from build123d import *

# Parameters (mm, degrees)
SKETCH1_R           = 4
BOSS_EXTRUDE1_DEPTH = 8.9
SKETCH2_R           = 5
BOSS_EXTRUDE2_DEPTH = 1.5
BOSS_EXTRUDE3_START = -1.5
SKETCH3_R           = 40
BOSS_EXTRUDE3_DEPTH = 3
CUT_EXTRUDE2_START  = 8.9
SKETCH5_R           = 2.2
CUT_EXTRUDE2_DEPTH  = 2
CUT_EXTRUDE3_DEPTH  = 10


with BuildPart() as part:
    # Sketch1 → Boss-Extrude1 (new body)
    with BuildSketch(Plane.XY):
        Circle(SKETCH1_R)
    extrude(amount=BOSS_EXTRUDE1_DEPTH)

    # Sketch2 → Boss-Extrude2 (add)
    with BuildSketch(Plane.XY):
        Circle(SKETCH2_R)
    extrude(amount=-BOSS_EXTRUDE2_DEPTH)

    # Sketch3 → Boss-Extrude3 (add)
    with BuildSketch(Plane.XY.offset(BOSS_EXTRUDE3_START)):
        Circle(SKETCH3_R)
    extrude(amount=-BOSS_EXTRUDE3_DEPTH)

    # Sketch5 → Cut-Extrude2 (cut)
    with BuildSketch(Plane.XY.offset(CUT_EXTRUDE2_START)):
        Circle(SKETCH5_R)
    extrude(amount=-CUT_EXTRUDE2_DEPTH, mode=Mode.SUBTRACT)

    # Sketch6 → Cut-Extrude3 (cut)
    with BuildSketch(Plane.XY):
        with BuildLine():
            Line((30.266810214, -15.165149948), (8.5033321, -2.6))
            ThreePointArc((8.5033321, -2.6), (7.973884535, -2.083913954), (7.755291283, -1.377602039))
            ThreePointArc((7.755291283, -1.377602039), (8, 0), (7.755291283, 1.377602039))
            ThreePointArc((7.755291283, 1.377602039), (7.973884535, 2.083913954), (8.5033321, 2.6))
            Line((8.5033321, 2.6), (30.266810214, 15.165149948))
            ThreePointArc((30.266810214, 15.165149948), (31.724798793, 15.379954672), (32.934114256, 14.537679256))
            ThreePointArc((32.934114256, 14.537679256), (36, 0), (32.934114256, -14.537679256))
            ThreePointArc((32.934114256, -14.537679256), (31.724798793, -15.379954672), (30.266810214, -15.165149948))
        make_face()
        with BuildLine():
            Line((2, 33.794401511), (2, 8.664101615))
            ThreePointArc((2, 8.664101615), (2.182219844, 7.947543551), (2.684607279, 7.405080285))
            ThreePointArc((2.684607279, 7.405080285), (4, 6.92820323), (5.070684004, 6.027478245))
            ThreePointArc((5.070684004, 6.027478245), (5.791664691, 5.863629597), (6.5033321, 6.064101615))
            Line((6.5033321, 6.064101615), (28.266810214, 18.629251563))
            ThreePointArc((28.266810214, 18.629251563), (29.181830852, 19.784504349), (29.057056676, 21.252939969))
            ThreePointArc((29.057056676, 21.252939969), (18, 31.176914536), (3.87705758, 35.790619225))
            ThreePointArc((3.87705758, 35.790619225), (2.542967941, 35.164459021), (2, 33.794401511))
        make_face()
        with BuildLine():
            Line((2, -33.794401511), (2, -8.664101615))
            ThreePointArc((2, -8.664101615), (2.182219844, -7.947543551), (2.684607279, -7.405080285))
            ThreePointArc((2.684607279, -7.405080285), (4, -6.92820323), (5.070684004, -6.027478245))
            ThreePointArc((5.070684004, -6.027478245), (5.791664691, -5.863629597), (6.5033321, -6.064101615))
            Line((6.5033321, -6.064101615), (28.266810214, -18.629251563))
            ThreePointArc((28.266810214, -18.629251563), (29.181830852, -19.784504349), (29.057056676, -21.252939969))
            ThreePointArc((29.057056676, -21.252939969), (18, -31.176914536), (3.87705758, -35.790619225))
            ThreePointArc((3.87705758, -35.790619225), (2.542967941, -35.164459021), (2, -33.794401511))
        make_face()
        with BuildLine():
            Line((-28.266810214, -18.629251563), (-6.5033321, -6.064101615))
            ThreePointArc((-6.5033321, -6.064101615), (-5.791664691, -5.863629597), (-5.070684004, -6.027478245))
            ThreePointArc((-5.070684004, -6.027478245), (-4, -6.92820323), (-2.684607279, -7.405080285))
            ThreePointArc((-2.684607279, -7.405080285), (-2.182219844, -7.947543551), (-2, -8.664101615))
            Line((-2, -8.664101615), (-2, -33.794401511))
            ThreePointArc((-2, -33.794401511), (-2.542967941, -35.164459021), (-3.87705758, -35.790619225))
            ThreePointArc((-3.87705758, -35.790619225), (-18, -31.176914536), (-29.057056676, -21.252939969))
            ThreePointArc((-29.057056676, -21.252939969), (-29.181830852, -19.784504349), (-28.266810214, -18.629251563))
        make_face()
        with BuildLine():
            Line((-30.266810214, 15.165149948), (-8.5033321, 2.6))
            ThreePointArc((-8.5033321, 2.6), (-7.973884535, 2.083913954), (-7.755291283, 1.377602039))
            ThreePointArc((-7.755291283, 1.377602039), (-8, 0), (-7.755291283, -1.377602039))
            ThreePointArc((-7.755291283, -1.377602039), (-7.973884535, -2.083913954), (-8.5033321, -2.6))
            Line((-8.5033321, -2.6), (-30.266810214, -15.165149948))
            ThreePointArc((-30.266810214, -15.165149948), (-31.724798793, -15.379954672), (-32.934114256, -14.537679256))
            ThreePointArc((-32.934114256, -14.537679256), (-36, 0), (-32.934114256, 14.537679256))
            ThreePointArc((-32.934114256, 14.537679256), (-31.724798793, 15.379954672), (-30.266810214, 15.165149948))
        make_face()
        with BuildLine():
            Line((-2, 33.794401511), (-2, 8.664101615))
            ThreePointArc((-2, 8.664101615), (-2.182219844, 7.947543551), (-2.684607279, 7.405080285))
            ThreePointArc((-2.684607279, 7.405080285), (-4, 6.92820323), (-5.070684004, 6.027478245))
            ThreePointArc((-5.070684004, 6.027478245), (-5.791664691, 5.863629597), (-6.5033321, 6.064101615))
            Line((-6.5033321, 6.064101615), (-28.266810214, 18.629251563))
            ThreePointArc((-28.266810214, 18.629251563), (-29.181830852, 19.784504349), (-29.057056676, 21.252939969))
            ThreePointArc((-29.057056676, 21.252939969), (-18, 31.176914536), (-3.87705758, 35.790619225))
            ThreePointArc((-3.87705758, 35.790619225), (-2.542967941, 35.164459021), (-2, 33.794401511))
        make_face()
    extrude(amount=-CUT_EXTRUDE3_DEPTH, mode=Mode.SUBTRACT)


solid = part.part
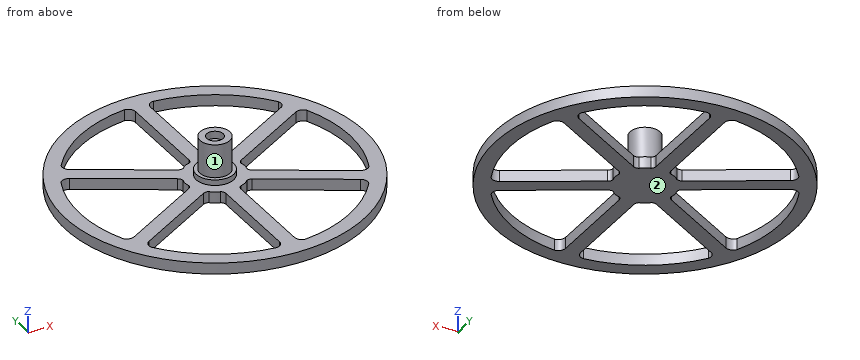
Work out the finished part from the listing and answer in its coordinate system (mm). Face numbers are marked on the shaded views. A direction names the side the tool comes from. Round coordinates to 2 decimals unless told otherwise and drop trailing zeros. Loops run counter-clockwise (first coordinate to the right, second up) from the corner with the lowest first, then second, coordinate; pieces in that order, holes last. Notation, with made-up numbers: (-5.5, -5) - (20.5, -5) arc R23 cw to (20.5, 4) - close; hole circle Ø3 at (87, 13.5). An arc over 180 degrees is marked (long way). One line per item, written item: value.
Q1. Find section C-C on y = 13. Give the vertices of the cut face in (x, z), and give its area (3 significant figures).
Check values:
outline: (-37.83, -4.5) - (-33.57, -4.5) - (-33.57, -1.5) - (-37.83, -1.5) - close; (-26.52, -4.5) - (-18.52, -4.5) - (-18.52, -1.5) - (-26.52, -1.5) - close; (-2, -4.5) - (2, -4.5) - (2, -1.5) - (-2, -1.5) - close; (18.52, -4.5) - (26.52, -4.5) - (26.52, -1.5) - (18.52, -1.5) - close; (33.57, -4.5) - (37.83, -4.5) - (37.83, -1.5) - (33.57, -1.5) - close
area: 85.5 mm2
Q2. Find section D-D on x = -10. Give the vertices of the cut face in (y, z), and give its area (3 significant figures).
Check values:
outline: (-38.73, -4.5) - (-34.58, -4.5) - (-34.58, -1.5) - (-38.73, -1.5) - close; (-8.08, -4.5) - (-3.46, -4.5) - (-3.46, -1.5) - (-8.08, -1.5) - close; (3.46, -4.5) - (8.08, -4.5) - (8.08, -1.5) - (3.46, -1.5) - close; (34.58, -4.5) - (38.73, -4.5) - (38.73, -1.5) - (34.58, -1.5) - close
area: 52.6 mm2
Q3. Each of these flat-tipped pins is pushed along its axis until it touches: pin 1 Ø3 at (y, z) = (7.5, 2) entering from -X; pin 2 Ø3 at (x, y) = (-3, -20) entering from +Z; pin 3 Ø2.5 at (y, z) = (-15.5, -3) entering from +X; pin 4 Ø3.5 at (y, z) = (26.5, -3.5) entering from +X. Where does it stop, or does it pass through?
Check values:
pin 1: through
pin 2: z = -1.5
pin 3: x = 37.38
pin 4: x = 31.42
Q4. For the marked faces 1 and 2, determine the directions among +Z, -Z, +X, -X, +Y, -Y from which every point of the face is accessible in a straight line to the end or side of a thin tool.
Check values:
face 1: +Z
face 2: -Z, +X, -X, +Y, -Y
Q5. Straight lines are drawn through the part: probe 1 along Y at (x, z) = (-22, -3.5); probe 2 along Z at (x, y) = (9.5, -7.5); probe 3 along Y at (x, z) = (20.5, -3.75). For each, find the intervals that lie inside material, in ascending order.
Check values:
probe 1: -33.41 to -28.5, -15.01 to -10.39, 10.39 to 15.01, 28.5 to 33.41
probe 2: -4.5 to -1.5
probe 3: -34.35 to -29.59, -14.15 to -9.53, 9.53 to 14.15, 29.59 to 34.35
Q6. Find section A-A on y = 0. Give the vertices of the cut face in (x, z), and give its area (3 significant figures).
Check values:
outline: (-40, -4.5) - (-36, -4.5) - (-36, -1.5) - (-40, -1.5) - close; (-8, -4.5) - (8, -4.5) - (8, -1.5) - (5, -1.5) - (5, 0) - (4, 0) - (4, 8.9) - (2.2, 8.9) - (2.2, 6.9) - (-2.2, 6.9) - (-2.2, 8.9) - (-4, 8.9) - (-4, 0) - (-5, 0) - (-5, -1.5) - (-8, -1.5) - close; (36, -4.5) - (40, -4.5) - (40, -1.5) - (36, -1.5) - close
area: 149 mm2
Q7. Find section B-B on x = 0. Give the vertices of the cut face in (y, z).
Check values:
outline: (-40, -4.5) - (40, -4.5) - (40, -1.5) - (5, -1.5) - (5, 0) - (4, 0) - (4, 8.9) - (2.2, 8.9) - (2.2, 6.9) - (-2.2, 6.9) - (-2.2, 8.9) - (-4, 8.9) - (-4, 0) - (-5, 0) - (-5, -1.5) - (-40, -1.5) - close
